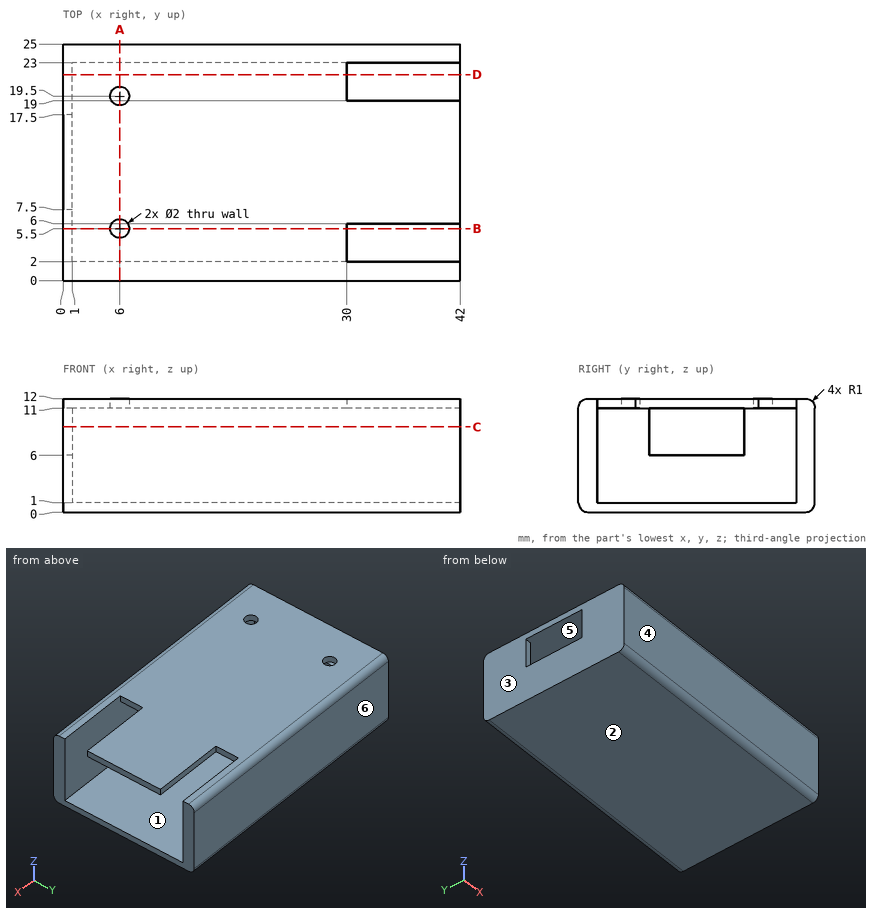
Verification items for this drawing (mm, ordinates from the low corner). A direction names the side the tool comes from. Give positions to 0.01 mm unless a question says otherwise; leave off trailing zeros. Loops run counter-clockwise (first coordinate to the right, second up) from the corner with the lowest first, then second, coordinate; pieces in that order, holes last. Notation, with made-up numbers: M 89,-32 L 128,-32 A17 cw 128,1 Z; hole C -19,-36.75 d1. An arc over 180 degrees is marked long. Answer in a Markdown table with one row per item.
1) Mould release check, pull along Y, two halves, no side actions. Record for the marked faces 3, 4, 5 and 6: released by +Y, released by -Y, zero draft, split by the parting line, or undercut.
Solutions:
| item | result |
|---|---|
| face 3 | zero draft |
| face 4 | released by -Y |
| face 5 | undercut |
| face 6 | released by +Y |
2) Thickness scan on line 1 (Z direction, x = 38, y = 12.5); line 2 (Y direction, x = 7, z = 1.25); line 3 (Y direction, x = 6, z = 11.55). Record the ranges inside material, lowest first.
Solutions:
| item | result |
|---|---|
| line 1 | z = 0 to 1, 11 to 12 |
| line 2 | y = 0 to 2, 23 to 25 |
| line 3 | y = 0.16 to 4.5, 6.5 to 18.5, 20.5 to 24.84 |
3) Cross-section at A-A (x = 6). Enter the section's corners in (y, z), plus the area to 3 significant figures.
Solutions:
| item | result |
|---|---|
| outline | M 0,1 A1 ccw 1,0 L 24,0 A1 ccw 25,1 L 25,11 A1 ccw 24,12 L 20.5,12 L 20.5,11 L 23,11 L 23,1 L 2,1 L 2,11 L 4.5,11 L 4.5,12 L 1,12 A1 ccw 0,11 Z; M 6.5,11 L 18.5,11 L 18.5,12 L 6.5,12 Z |
| area | 85.1 mm^2 |
4) Tool access check on the marked faces 1 and 2. Record the directions out of +Z, -Z, +X, -X, +Y, -Y that give a thin tool (end or side, any length) a straight path to the whole face; none if there is none.
Solutions:
| item | result |
|---|---|
| face 1 | +X |
| face 2 | -Z, +X, -X, +Y, -Y |
5) Depth check by flat-ended pin: pin 1 (5 mm diameter, centred on y = 15.5, z = 6.5, fed in from +X); pin 2 (1.1 mm diameter, centred on y = 21, z = 11.5, fed in from +X); pin 3 (1.8 mm diameter, centred on x = 6, y = 19.5, fed in from +Z). Enter the tip coordinate at first touch or a pass-through.
Solutions:
| item | result |
|---|---|
| pin 1 | stops at x = 1 |
| pin 2 | stops at x = 30 |
| pin 3 | stops at z = 1 |
6) Cross-section at B-B (y = 5.5). Enter the section's corners in (x, z), plus the area to 3 significant figures.
Solutions:
| item | result |
|---|---|
| outline | M 0,0 L 42,0 L 42,1 L 1,1 L 1,11 L 5,11 L 5,12 L 0,12 Z; M 7,11 L 30,11 L 30,12 L 7,12 Z |
| area | 80.0 mm^2 |
7) Cross-section at D-D (y = 21.75). Enter the section's corners in (x, z).
Solutions:
| item | result |
|---|---|
| outline | M 0,0 L 42,0 L 42,1 L 1,1 L 1,11 L 30,11 L 30,12 L 0,12 Z |
8) Cross-section at C-C (z = 9). Enter the section's corners in (x, y), plus the area to 3 significant figures.
Solutions:
| item | result |
|---|---|
| outline | M 0,0 L 42,0 L 42,2 L 1,2 L 1,7.5 L 0,7.5 Z; M 0,17.5 L 1,17.5 L 1,23 L 42,23 L 42,25 L 0,25 Z |
| area | 179 mm^2 |
